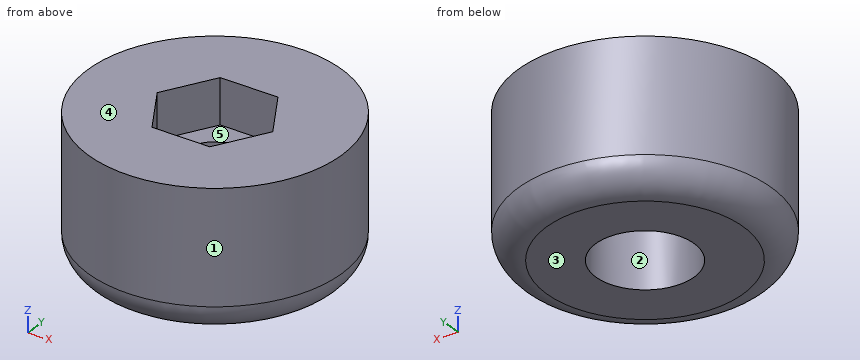
Autodesk Fusion 360 part; units mm, degrees
ref_plane "WorkPlane1" through (0, 0, 0) normal (0, 0, 1) x (1, 0, 0)
sketch "Sketch1" plane through (0, 0, 0) normal (0, 0, 1) x (1, 0, 0)
  circle A0 centre (0, 0) radius 9
  dimension "d2" = 18
extrude "Extrude1" add sketch "Sketch1" along normal blind 10
sketch "Sketch2" plane through (0, 0, 10) normal (0, 0, 1) x (-1, 0, 0)
  circle A0 centre (0, 0) radius 9
  line L0 (-2.0496, -3.55) -> (2.0496, -3.55)
  line L1 (2.0496, -3.55) -> (4.0992, 0)
  line L2 (4.0992, 0) -> (2.0496, 3.55)
  line L3 (2.0496, 3.55) -> (-2.0496, 3.55)
  line L4 (-2.0496, 3.55) -> (-4.0992, 0)
  line L5 (-4.0992, 0) -> (-2.0496, -3.55)
  dimension "d5" = 3.55
extrude "Extrude2" cut sketch "Sketch2" against normal blind 3.2 contours L0 L1 L2 L3 L4 L5
sketch "Sketch3" plane through (0, 0, 0) normal (0, 0, -1) x (1, 0, 0)
  circle A0 centre (0, 0) radius 9
  circle A1 centre (0, 0) radius 3.5
  dimension "d8" = 7
extrude "Extrude3" cut sketch "Sketch3" against normal blind 4.2 contours A1
sketch "Sketch4" plane through (0, 0, 4.2) normal (0, 0, -1) x (1, 0, 0)
  circle A0 centre (0, 0) radius 3.5
  circle A1 centre (0, 0) radius 2.1
  dimension "d11" = 4.2
extrude "Extrude4" cut sketch "Sketch4" against normal up to surface (2.6 mm away) contours A1
fillet "Fillet1" radius 2 1 edges at (-8.3909, -3.2545, 0)
equation "d5 = ( 7.1 / 2 ) * 1 mm"
Verification items for the finished model (mm, model axes). Face numbers are marked on the shaded views. A direction names the side the tool comes from. Coordinates: 2 decimals unless noted, no trailing zeros. Loops run counter-clockwise (first coordinate to the right, second up) from the corner with the lowest first, then second, coordinate; pieces in that order, holes last. Notation, with made-up numbers: (-25, 50) - (-6, 50) arc R35 cw to (-6, 87) - close; hole circle Ø2 at (-38.75, -34.5). An arc over 180 degrees is marked (long way). Answer as a JSON object with one key per item and string values.
(1) Access from +Z, -Z, +X, -X, +Y, -Y to the whole of each face (thin tool, end or side, straight path). Record for the marked faces 4 and 5.
Response:
{"face 4": "+Z, +X, -X, +Y, -Y", "face 5": "+Z"}
(2) Mould release check, pull along X, two halves, no side actions. Record for the marked faces 1, 2 and 3: pulls with the +X half, pulls with the -X half, needs draft (parallel to the pull), parting line crosses it, or undercut.
Response:
{"face 1": "parting line crosses it", "face 2": "undercut", "face 3": "needs draft"}
(3) Scan lines: line 1 along Y through (x, z) = (0, 2.15); line 2 along Y through (x, z) = (0, 6.35); line 3 along X through (y, z) = (0.5, 1). Record each from-to range of solid material in increasing order.
Response:
{"line 1": "y = -9 to -3.5, 3.5 to 9", "line 2": "y = -9 to -2.1, 2.1 to 9", "line 3": "x = -8.72 to -3.46, 3.46 to 8.72"}
(4) Cross-section at C-C, the plane z = 2.25. Record the boundary of the cut face in (x, y), then the cut area to 3 significant figures.
Response:
{"outline": "circle Ø18 at (0, 0); hole circle Ø7 at (0, 0)", "area": "216 mm²"}
(5) Cross-section at B-B, the plane z = 8.5. Record the boundary of the cut face in (x, y), then the cut area to 3 significant figures.
Response:
{"outline": "circle Ø18 at (0, 0); hole (-4.1, 0) - (-2.05, -3.55) - (2.05, -3.55) - (4.1, 0) - (2.05, 3.55) - (-2.05, 3.55) - close", "area": "211 mm²"}
(6) Go/stop test with flat-tipped pins: pin 1 Ø1 at (x, y) = (-5, 1.5) entering from -Z; pin 2 Ø2 at (x, y) = (-1, 0) entering from -Z; pin 3 Ø6 at (y, z) = (-5, 2.5) entering from -X; pin 4 Ø2 at (x, z) = (2, 2.5) entering from +Y. Record where each tip stops, or that it passes through.
Response:
{"pin 1": "stops at z = 0", "pin 2": "passes through", "pin 3": "stops at x = -8.77", "pin 4": "stops at y = 8.94"}
(7) Cross-section at A-A, the plane x = 0. Record the boundary of the cut face in (y, z).
Response:
{"outline": "(-9, 2) arc R2 ccw to (-7, 0) - (-3.5, 0) - (-3.5, 4.2) - (-2.1, 4.2) - (-2.1, 6.8) - (-3.55, 6.8) - (-3.55, 10) - (-9, 10) - close; (2.1, 4.2) - (3.5, 4.2) - (3.5, 0) - (7, 0) arc R2 ccw to (9, 2) - (9, 10) - (3.55, 10) - (3.55, 6.8) - (2.1, 6.8) - close"}
